Build history of the part. All positions in model axes, mm. Face numbers are marked on the shaded views. A direction names the side the tool comes from. Coordinates: 2 decimals unless noted, no trailing zeros. Loops run counter-clockwise (first coordinate to the right, second up) from the corner with the lowest first, then second, coordinate; pieces in that order, holes last. Notation, with made-up numbers: M 47,7 L 103,7 A20 cw 103,41 Z; hole C 22,80.25 d11. An arc over 180 degrees is marked long. Write each question's results on one line, items separated by ' | '. Start each with the question number.
from build123d import *

# Parameters (mm, degrees)
SKETCH1_W               = 20
SKETCH1_H               = 20
BOSS_EXTRUDE1_DEPTH     = 20
SKETCH2_W               = 16.5
SKETCH2_H               = 16
CUT_EXTRUDE1_DEPTH      = 16.5
CUT_EXTRUDE2_DEPTH      = 34.526109228
CUT_EXTRUDE2_DEPTH_BACK = 34.526109228
CUT_EXTRUDE3_DEPTH      = 33.74522866
CUT_EXTRUDE3_DEPTH_BACK = 33.74522866
SKETCH4_R               = 2.5
CUT_EXTRUDE4_DEPTH      = 33.74522866
CUT_EXTRUDE4_DEPTH_BACK = 33.74522866
SKETCH5_R               = 2.5


with BuildPart() as part:
    # Sketch1 → Boss-Extrude1 (new body)
    with BuildSketch(Plane(origin=(0, 0, 0), x_dir=(1, 0, 0), z_dir=(0, 1, 0))):
        with Locations((-10, 10)):
            Rectangle(SKETCH1_W, SKETCH1_H)
    extrude(amount=BOSS_EXTRUDE1_DEPTH)

    # Sketch2 → Cut-Extrude1 (cut)
    with BuildSketch(Plane.ZY.offset(20)):
        with Locations((-8.25, 10)):
            Rectangle(SKETCH2_W, SKETCH2_H)
    extrude(amount=-CUT_EXTRUDE1_DEPTH, mode=Mode.SUBTRACT)

    # Sketch3 → Cut-Extrude2 (cut, two sides: drawn at the far end of the back side and taken through both)
    with BuildSketch(Plane(origin=(0, 18, 0), x_dir=(-1, 0, 0), z_dir=(0, -1, 0)).offset(-CUT_EXTRUDE2_DEPTH_BACK)):
        Polygon((63.738492046, 60.238492046), (20, 16.5), (3.5, 0), (-40.238492046, -43.738492046), (47.238492046, -131.215476139), (151.215476139, -27.238492046), align=None)
    extrude(amount=CUT_EXTRUDE2_DEPTH + CUT_EXTRUDE2_DEPTH_BACK, mode=Mode.SUBTRACT)

    # Sketch4 → Cut-Extrude3 (cut, two sides: drawn at the far end of the back side and taken through both)
    with BuildSketch(Plane.ZY.offset(3.5).offset(-CUT_EXTRUDE3_DEPTH_BACK)):
        with Locations((-7.5, 10)):
            Circle(SKETCH4_R)
    extrude(amount=CUT_EXTRUDE3_DEPTH + CUT_EXTRUDE3_DEPTH_BACK, mode=Mode.SUBTRACT)

    # Sketch5 → Cut-Extrude4 (cut, two sides: drawn at the far end of the back side and taken through both)
    with BuildSketch(Plane.XY.offset(-16.5).offset(-CUT_EXTRUDE4_DEPTH_BACK)):
        with Locations((-12.5, 10)):
            Circle(SKETCH5_R)
    extrude(amount=CUT_EXTRUDE4_DEPTH + CUT_EXTRUDE4_DEPTH_BACK, mode=Mode.SUBTRACT)


solid = part.part
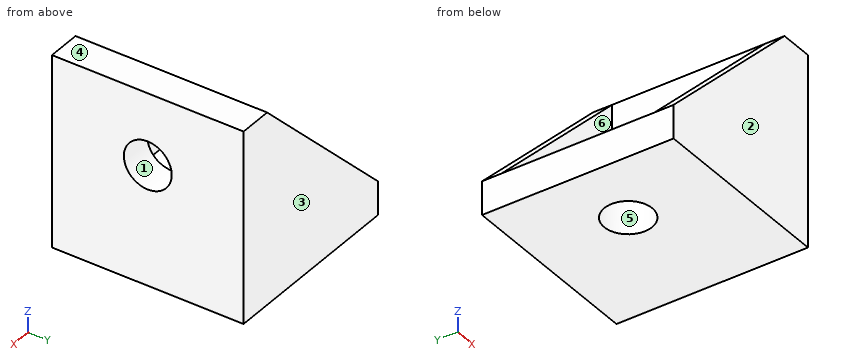
1. Band-saw the part on A-A, the plane y = 10. List the corners of the cut face in (x, z), plus the area to 4 significant figures.
2. Band-saw the part on C-C, the plane z = -9. List the corners of the cut face in (x, y), plus the area to 3 significant figures.
3. Pin check, flat tips, straight feed: pin 1 (4.5 mm diameter, centred on x = -12.5, y = 10, fed in from -Z); pin 2 (2 mm diameter, centred on x = -11.5, y = 7, fed in from +Z); pin 3 (5 mm diameter, centred on x = -11.5, y = 3.5, fed in from +Z); pin 4 (8 mm diameter, centred on y = 9.5, z = -9, fed in from -X). Stop position of each tip, or through.
4. Wall check: line 1 along X through (y, z) = (10, -18.9); line 2 along Y through (x, z) = (-1.55, -7.5); line 3 along Z through (x, y) = (-2.2, 10). Give the ranges that are in metal, low to high.
5. Band-saw the part on B-B, the plane x = -12.5. List the corners of the cut face in (y, z).
6. Mould opens along Y. For the marked faces 1, 2, 3 and 4 say: +Y half, -Y half, draft (parallel to the pull), parting line (faces both ways), or undercut.
7. Which spindle directions (+Z, -Z, +X, -X, +Y, -Y) get a long thin tool onto all of the face, cutting with end or side? Do the marked faces 5 and 6. Say none if no direction does.
8. Band-saw the part on D-D, the plane x = -4.25. List the corners of the cut face in (y, z).
Checked values:
1) outline: M -20,-20 L -15,-20 L -15,-16.5 L -20,-16.5 Z; M -10,-20 L 0,-20 L 0,-10 L -3.5,-10 L -3.5,-16.5 L -10,-16.5 Z; M -3.5,-5 L 0,-5 L 0,0 L -3.5,0 Z | area: 92.75 mm²
2) outline: M -12.5,0 L 0,0 L 0,8 L -3.5,8 L -3.5,2 L -12.5,2 Z; M -12.5,18 L -3.5,18 L -3.5,12 L 0,12 L 0,20 L -12.5,20 Z | area: 92.0 mm²
3) pin 1: through | pin 2: z = -16.5 | pin 3: z = -6 | pin 4: x = -3.5
4) line 1: -20 to -15, -10 to 0 | line 2: 0 to 7.5, 12.5 to 20 | line 3: -20 to -10, -5 to 0
5) outline: M 0,-20 L 7.5,-20 L 7.5,-16.5 L 2,-16.5 L 2,-9 L 0,-9 Z; M 12.5,-20 L 20,-20 L 20,-9 L 18,-9 L 18,-16.5 L 12.5,-16.5 Z
6) face 1: undercut | face 2: -Y half | face 3: +Y half | face 4: draft
7) face 5: +Z, -Z | face 6: +Z, -X
8) outline: M 0,-20 L 20,-20 L 20,-0.75 L 18,-0.75 L 18,-16.5 L 2,-16.5 L 2,-0.75 L 0,-0.75 Z
